from build123d import *

# Parameters (mm, degrees)
BOSS_EXTRUDE2_DEPTH = 3
BOSS_EXTRUDE3_DEPTH = 50


with BuildPart() as part:
    # Sketch1 → Boss-Extrude2 (new body)
    # profile 1 of 2: a face of its own
    with BuildSketch(Plane(origin=(0, 0, 0), x_dir=(1, 0, 0), z_dir=(0, 1, 0))):
        Polygon((23.212466677, -13.401723884), (23.212466677, 13.401723884), (0, 26.803447769), (-23.212466677, 13.401723884), (-23.212466677, -13.401723884), (0, -26.803447769), align=None)
        Polygon((21.212466677, -12.247023346), (21.212466677, 12.247023346), (0, 24.494046692), (-21.212466677, 12.247023346), (-21.212466677, -12.247023346), (0, -24.494046692), align=None, mode=Mode.SUBTRACT)
    # profile 2 of 2: a face of its own
    with BuildSketch(Plane(origin=(0, 0, 0), x_dir=(1, 0, 0), z_dir=(0, 1, 0))):
        Polygon((0, -24.494046692), (21.212466677, -12.247023346), (21.212466677, 12.247023346), (0, 24.494046692), (-21.212466677, 12.247023346), (-21.212466677, -12.247023346), align=None)
    extrude(amount=BOSS_EXTRUDE2_DEPTH)

    # Sketch1_4 → Boss-Extrude3 (add)
    with BuildSketch(Plane(origin=(0, 0, 0), x_dir=(1, 0, 0), z_dir=(0, 1, 0))):
        Polygon((0, 26.803447769), (-23.212466677, 13.401723884), (-23.212466677, -13.401723884), (0, -26.803447769), (23.212466677, -13.401723884), (23.212466677, 13.401723884), align=None)
        Polygon((21.212466677, 12.247023346), (0, 24.494046692), (-21.212466677, 12.247023346), (-21.212466677, -12.247023346), (0, -24.494046692), (21.212466677, -12.247023346), align=None, mode=Mode.SUBTRACT)
    extrude(amount=BOSS_EXTRUDE3_DEPTH)


solid = part.part
Work out the finished part from the listing and answer in its coordinate system (mm). A direction names the side the tool comes from. Give positions to 0.01 mm unless a question says otherwise; leave off trailing zeros. Order: outer loops, then holes, each group sorted by start corner. A loop starts at its lowest first (then second) coordinate and runs counter-clockwise, first axis right, second up. Notation, with made-up numbers: (74.25, -14) - (116.25, -14) arc R12 ccw to (116.25, 7) - close; hole circle Ø11 at (-6, 80.5). An arc over 180 degrees is marked (long way). Answer as CSV lines item,"result". Start each with the question number.
Q1. The part is cut by section B-B (x = 17). Write down the section's boundary in (y, z).
Q2. Find the intervals of material crossed by L1, parallel to X at y = 33.5, z = 2.5; L2, parallel to Z at x = 0, y = 40; L3, parallel to Y at x = -15, z = 11, in increasing order. Write a range as [from, to].
Q3. Given pin 1 Ø1.5 at (x, y) = (-7, 10) entering from -Z (3 decimals); pin 2 Ø5 at (x, y) = (18, 30) entering from +Z; pin 3 Ø5 at (x, z) = (2.5, -11.5) entering from +Y; pin 4 Ø12 at (y, z) = (17, 16.5) entering from +X, each flat-ended and moving along its own axis, determine where each tip first touches the part or whether it passes through.
Q4. The part is cut by section A-A (y = 4). Write down the section's boundary in (x, z), then the cut area to 3 significant figures.
Q5. The mould has two halves that part along X. Classify faces 3 (the face through (21.212, 26, 0)), 4 (the face through (11.44, 24.65, 20.2)), 5 (the face through (-11.77, 24.65, 20.01)): +X half, -X half, draft (parallel to the pull), parting line (faces both ways), or undercut.
Q6. The part is cut by section C-C (z = 15.5). Write down the section's boundary in (x, y).
Q7. For faces 1 (the face through (23.212, 25, 0)), 2 (the face through (-21.212, 26, 0)), determine the directions among +Z, -Z, +X, -X, +Y, -Y from which every point of the face is accessible in a straight line to the end or side of a thin tool.
Check result:
1,outline,"(0, -16.99) - (50, -16.99) - (50, -14.68) - (3, -14.68) - (3, 14.68) - (50, 14.68) - (50, 16.99) - (0, 16.99) - close"
2,L1,"x = [-23.21, -21.21], [21.21, 23.21]"
2,L2,"z = [-26.8, -24.49], [24.49, 26.8]"
2,L3,"y = [0, 3]"
3,pin 1,"stops at z = -23.195"
3,pin 2,"stops at z = 17.85"
3,pin 3,"stops at y = 3"
3,pin 4,"stops at x = 23.21"
4,outline,"(-23.21, -13.4) - (0, -26.8) - (23.21, -13.4) - (23.21, 13.4) - (0, 26.8) - (-23.21, 13.4) - close; hole (-21.21, -12.25) - (0, -24.49) - (21.21, -12.25) - (21.21, 12.25) - (0, 24.49) - (-21.21, 12.25) - close"
4,area,"308 mm²"
5,face 3,"undercut"
5,face 4,"+X half"
5,face 5,"-X half"
6,outline,"(-19.58, 0) - (19.58, 0) - (19.58, 50) - (15.58, 50) - (15.58, 3) - (-15.58, 3) - (-15.58, 50) - (-19.58, 50) - close"
7,face 1,"+Z, -Z, +X, +Y, -Y"
7,face 2,"+Y"
